Verification items for the finished model (mm, model axes). Give positions to 0.01 mm unless a question says otherwise; leave off trailing zeros. Order: outer loops, then holes, each group sorted by start corner. A loop starts at its lowest first (then second) coordinate and runs counter-clockwise, first axis right, second up.
from build123d import *

# Parameters (mm, degrees)
SKETCH1_R           = 6
BOSS_EXTRUDE1_DEPTH = 2
SKETCH2_R           = 5
BOSS_EXTRUDE2_DEPTH = 6
SKETCH3_R           = 6
BOSS_EXTRUDE3_DEPTH = 2
FILLET1_R           = 3
SKETCH4_R           = 1.8
CUT_EXTRUDE1_DEPTH  = 14.114877049


with BuildPart() as part:
    # Sketch1 → Boss-Extrude1 (new body)
    with BuildSketch(Plane(origin=(0, 0, 0), x_dir=(0, 0, -1), z_dir=(1, 0, 0))):
        Circle(SKETCH1_R)
    extrude(amount=BOSS_EXTRUDE1_DEPTH)

    # Sketch2 → Boss-Extrude2 (add)
    with BuildSketch(Plane(origin=(2, 0, 0), x_dir=(0, 0, -1), z_dir=(1, 0, 0))):
        Circle(SKETCH2_R)
    extrude(amount=BOSS_EXTRUDE2_DEPTH)

    # Sketch3 → Boss-Extrude3 (add)
    with BuildSketch(Plane(origin=(8, 0, 0), x_dir=(0, 0, -1), z_dir=(1, 0, 0))):
        Circle(SKETCH3_R)
    extrude(amount=BOSS_EXTRUDE3_DEPTH)

    # Fillet1
    # the kernel refuses this fillet: 3 mm, written as the material it adds along each edge
    with BuildSketch(Plane(origin=(2, 0, 0), x_dir=(0, 0, -1), z_dir=(0, -1, 0))) as fillet1_piece_1:
        with BuildLine():
            CenterArc((8, 2.236067977), FILLET1_R, 180, 48.189685104)
            Line((6, 0), (5.96, -0.04472136))
            ThreePointArc((5.96, -0.04472136), (5.5, -0.06), (5, -0.06))
            Line((5, -0.06), (4.94, 0))
            Line((4.94, 0), (4.94, 2.236067977))
            Line((4.94, 2.236067977), (5, 2.236067977))
        make_face()
    revolve(axis=Axis((2, 0, 0), (1, 0, 0)))
    with BuildSketch(Plane(origin=(8, 0, 0), x_dir=(0, 0, -1), z_dir=(0, -1, 0))) as fillet1_piece_2:
        with BuildLine():
            CenterArc((8, -2.236067977), FILLET1_R, 131.810314896, 48.189685104)
            Line((5, -2.236067977), (4.94, -2.236067977))
            Line((4.94, -2.236067977), (4.94, 0))
            Line((4.94, 0), (5, 0.06))
            ThreePointArc((5, 0.06), (5.5, 0.06), (5.96, 0.04472136))
            Line((5.96, 0.04472136), (6, 0))
        make_face()
    revolve(axis=Axis((8, 0, 0), (1, 0, 0)))

    # Sketch4 → Cut-Extrude1 (cut, through all)
    with BuildSketch(Plane.ZY):
        Circle(SKETCH4_R)
    extrude(amount=-CUT_EXTRUDE1_DEPTH, mode=Mode.SUBTRACT)


solid = part.part
(1) Section check C-C, the plane x = 7. Enter the section's corners in (y, z).
Solved:
outline: circle Ø10.53 at (0, 0); hole circle Ø3.6 at (0, 0)
(2) Section check A-A, the plane z = 0. Enter the section's corners in (x, y), then the cut area to 3 significant figures.
Solved:
outline: (0, -6) - (2, -6) arc R3 cw to (4.24, -5) - (5.76, -5) arc R3 cw to (8, -6) - (10, -6) - (10, -1.8) - (0, -1.8) - close; (0, 1.8) - (10, 1.8) - (10, 6) - (8, 6) arc R3 cw to (5.76, 5) - (4.24, 5) arc R3 cw to (2, 6) - (0, 6) - close
area: 74.7 mm2
(3) Go/stop test with flat-tipped pins: pin 1 (5 mm diameter, centred on x = 4.5, y = 1, fed in from -Z); pin 2 (2 mm diameter, centred on x = 5.5, y = -4.5, fed in from -Z); pin 3 (5 mm diameter, centred on x = 5.5, y = 1, fed in from +Z); pin 4 (2 mm diameter, centred on y = 0, z = 0, fed in from -X). Record where each tip stops, or that it passes through.
Solved:
pin 1: stops at z = -5.94
pin 2: stops at z = -3.57
pin 3: stops at z = 5.94
pin 4: passes through
(4) Scan lines: line 1 (Y direction, x = 5, z = 0); line 2 (X direction, y = 4.5, z = 2.75); line 3 (Y direction, x = 6.5, z = -0.25). Record each from-to range of solid material in increasing order.
Solved:
line 1: y = -5 to -1.8, 1.8 to 5
line 2: x = 0 to 2.98, 7.02 to 10
line 3: y = -5.09 to -1.78, 1.78 to 5.09
(5) Release check for a two-part mould opening along X. For faces 1 (the cylindrical face through (9, 0, 6)), 2 (the cylindrical face through (4.99, -4.88, 1.08)), 3 (the flat face through (10, 1.4, 1.4)) record: pulls with the +X half, pulls with the -X half, needs draft (parallel to the pull), parting line crosses it, or undercut.
Solved:
face 1: needs draft
face 2: undercut
face 3: pulls with the +X half
